For this review, use the dimensioned drawing (mm, ordinates from the lowest corner) and the shaded views. Round coordinates to 2 decimals unless told otherwise and drop trailing zeros. Write each loop counter-clockwise with the first axis right and the second up, starting at its lowest first coordinate (ties: lowest second). Pieces come first, ordered by that corner, then holes. Notation, with made-up numbers: M 53,6 L 91,6 A8 cw 91,14 Z; hole C -27.75,4 d8. An arc over 180 degrees is marked long. Write each question's results on one line, items separated by ' | '. Start each with the question number.
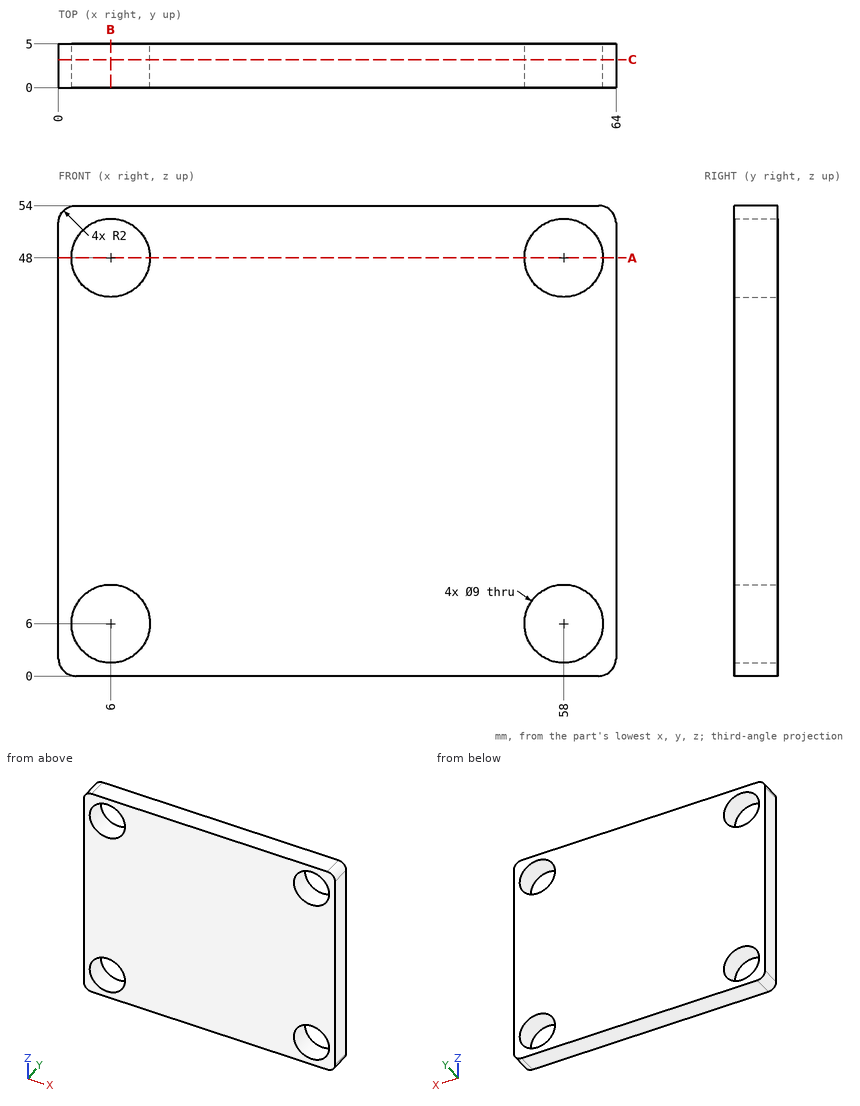
Item 1: We need section A-A on z = 48. State the section outline as (x, y) points.
Item 2: For probe 1 along X at (y, z) = (2.75, 48); probe 2 along Z at (x, y) = (6, 1.8); probe 3 along X at (y, z) = (0.95, 46), list the stretches that pass through material, from the lowest coordinate up.
Item 3: We need section C-C on y = 3.2. State the section outline as (x, z) points, then the cut area to 3 significant figures.
Item 4: Insertion check: P1, Ø7, axis at x = 58, z = 6, coming from the +Y side (3 decimals). The pin has a flat end and moves straight along its axis. Give the tip position at first contact, or say it passes through.
Item 5: We need section B-B on x = 6. State the section outline as (y, z) points, then the cut area to 3 significant figures.
Numbers:
1) outline: M 0,0 L 1.5,0 L 1.5,5 L 0,5 Z; M 10.5,0 L 53.5,0 L 53.5,5 L 10.5,5 Z; M 62.5,0 L 64,0 L 64,5 L 62.5,5 Z
2) probe 1: x = 0 to 1.5, 10.5 to 53.5, 62.5 to 64 | probe 2: z = 0 to 1.5, 10.5 to 43.5, 52.5 to 54 | probe 3: x = 0 to 1.97, 10.03 to 53.97, 62.03 to 64
3) outline: M 0,2 A2 ccw 2,0 L 62,0 A2 ccw 64,2 L 64,52 A2 ccw 62,54 L 2,54 A2 ccw 0,52 Z; hole C 6,6 d9; hole C 6,48 d9; hole C 58,6 d9; hole C 58,48 d9 | area: 3,200 mm^2
4) P1: passes through
5) outline: M 0,0 L 5,0 L 5,1.5 L 0,1.5 Z; M 0,10.5 L 5,10.5 L 5,43.5 L 0,43.5 Z; M 0,52.5 L 5,52.5 L 5,54 L 0,54 Z | area: 180 mm^2
